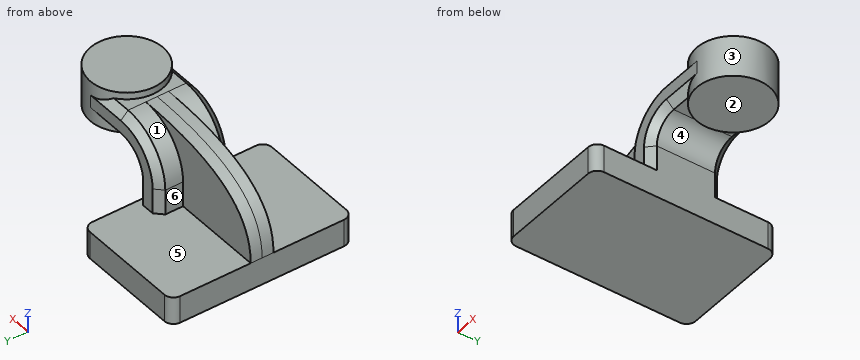
```python
from build123d import *

# Parameters (mm, degrees)
F1_DEPTH = 63.5
F0_W     = 25.4132496778
F0_H     = 19.05
F2_DEPTH = 25.4
F3_DEPTH = 7.9375
F5_R     = 6.35
F6_SIZE  = 5.08


with BuildPart() as f1:
    # F0 (on Front) → F1 (new body, symmetric)
    with BuildSketch(Plane.XZ):
        Polygon((41.275, -9.525), (41.275, 9.525), (22.225, 9.525), (-41.275, 9.525), (-41.275, -9.525), align=None)
    extrude(amount=F1_DEPTH, both=True)

    # F0 (on Front) → F2 (join, symmetric)
    with BuildSketch(Plane.XZ):
        with BuildLine():
            Line((22.225, 9.525), (41.275, 9.525))
            Line((41.275, 9.525), (41.275, 27.0002))
            ThreePointArc((41.275, 27.0002), (45.9246798487, 38.2255201513), (57.15, 42.8752))
            Line((57.15, 42.8752), (60.325, 42.8752))
            Line((60.325, 42.8752), (60.325, 61.9252))
            Line((60.325, 61.9252), (57.15, 61.9252))
            ThreePointArc((57.15, 61.9252), (32.4542956671, 51.6959043329), (22.225, 27.0002))
            Line((22.225, 27.0002), (22.225, 9.525))
        make_face()
        with Locations((73.0316248389, 52.4002)):
            Rectangle(F0_W, F0_H)
    extrude(amount=F2_DEPTH, both=True)

    # F0 (on Front) → F3 (join, symmetric)
    with BuildSketch(Plane.XZ):
        with BuildLine():
            Line((-41.275, 9.525), (22.225, 9.525))
            Line((22.225, 9.525), (22.225, 27.0002))
            ThreePointArc((22.225, 27.0002), (32.4542956671, 51.6959043329), (57.15, 61.9252))
            add(Edge.make_bspline(
                [(-41.275, 9.525), (-41.275, 49.0254089236), (0, 61.9252), (57.15, 61.9252)],
                knots=[0, 0, 0, 0, 111.5045361635, 111.5045361635, 111.5045361635, 111.5045361635], degree=3))
        make_face()
    extrude(amount=F3_DEPTH, both=True)

    # F0 (on Front) → F4 (revolve)
    with BuildSketch(Plane.XZ):
        Polygon((85.7382496778, 61.9252), (85.7382496778, 42.8752), (85.7382496778, 38.1), (111.125, 38.1), (111.125, 66.675), (85.7382496778, 66.675), align=None)
    revolve(axis=Axis((85.7382496778, 0, 52.3875), (0, 0, 1)))

    # F5
    f5_edges = [f1.edges().sort_by_distance(p)[0] for p in [
        (-41.275, -63.5, 0),
        (41.275, -63.5, 0),
        (41.275, 63.5, 0),
        (-41.275, 63.5, 0),
    ]]
    fillet(f5_edges, radius=F5_R)

    # F6
    f6_edges = [f1.edges().sort_by_distance(p)[0] for p in [
        (32.454296, 25.4, 51.695904),
        (32.454296, -25.4, 51.695904),
        (45.92468, -25.4, 38.22552),
        (45.92468, 25.4, 38.22552),
    ]]
    chamfer(f6_edges, length=F6_SIZE)


solid = f1.part
```
Check sheet for the modelled part. Datum: model origin and axes. Units: mm. Face numbers are marked on the shaded views. A direction names the side the tool comes from. Coordinates: 2 decimals unless noted, no trailing zeros. Loops run counter-clockwise (first coordinate to the right, second up) from the corner with the lowest first, then second, coordinate; pieces in that order, holes last.
1) Material ranges on probe 1 along Y at (x, z) = (35.5, 56); probe 2 along X at (y, z) = (-28, 8) (3 decimals); probe 3 along X at (y, z) = (1, 11.5) (3 decimals), recorded low to high.
2) Access from +Z, -Z, +X, -X, +Y, -Y to the whole of each face (thin tool, end or side, straight path). Record for the marked faces 1, 2 and 3.
3) Sectioned sample at A-A (y = -40). Record the boundary of the cut face in (x, z) (3 decimals), and give its area (3 significant figures).
4) Release check for a two-part mould opening along X. For the marked faces 4, 5 and 6 record: released by +X, released by -X, zero draft, split by the parting line, or undercut.
5) Sectioned sample at B-B (x = 90). Record the boundary of the cut face in (y, z) (3 decimals).
6) Gauge pin test, flat ends, axial feed: pin 1 (1.5 mm diameter, centred on x = 31, y = 1.5, fed in from +Z); pin 2 (14 mm diameter, centred on x = 49, z = 37.5, fed in from -Y); pin 3 (13.5 mm diameter, centred on y = 15, z = 21.5, fed in from -X) (3 decimals). Record the tip position at first contact, or that the pin passes through.
Check sheet entries:
1. probe 1: y = -7.94 to 7.94
1. probe 2: x = -41.275 to 41.275
1. probe 3: x = -41.24 to 41.275
2. face 1: +Z, -X, +Y
2. face 2: -Z, +X, +Y, -Y
2. face 3: none
3. outline: (-41.275, -9.525) - (41.275, -9.525) - (41.275, 9.525) - (-41.275, 9.525) - close
3. area: 1,570 mm2
4. face 4: undercut
4. face 5: zero draft
4. face 6: released by -X
5. outline: (-25.026, 38.1) - (25.026, 38.1) - (25.026, 66.675) - (-25.026, 66.675) - close
6. pin 1: stops at z = 60.94
6. pin 2: stops at y = -24.74
6. pin 3: stops at x = 22.225
